Input: dimensioned drawing with shaded views. Units: mm. Origin: part minimum x, y, z. A direction names the side the tool comes from. Round coordinates to 2 decimals unless told otherwise and drop trailing zeros. Loops run counter-clockwise (first coordinate to the right, second up) from the corner with the lowest first, then second, coordinate; pieces in that order, holes last.
1) Draft query along Y for the marked faces 1, 2 and 3. Return one class per face: pulls with the +Y half, pulls with the -Y half, needs draft (parallel to the pull), parting line crosses it, or undercut.
2) Section D-D, the plane z = 13. Return loops of the section in (x, y).
3) Ray query, line 1 along Y through (x, z) = (25, 19); line 2 along Z through (x, y) = (17.5, 81); line 3 along Y through (x, z) = (26, 29.5). Return the intervals inside material, ascending.
4) First-contact query: pin 1 (8 mm diameter, centred on x = 24.5, y = 78, fed in from +Z); pin 2 (11 mm diameter, centred on x = 25, y = 35, fed in from +Z); pin 3 (8 mm diameter, centred on x = 21.5, y = 52.5, fed in from -Z); pin 4 (3.5 mm diameter, centred on x = 12.5, z = 3.5, fed in from +Y). Flat tips, straight axial feed; report the tip coordinate or a pass-through.
5) Section A-A, the plane x = 25. Return loops of the section in (y, z).
6) Section C-C, the plane x = 18.5. Return loops of the section in (y, z).
7) Section B-B, the plane y = 35. Return loops of the section in (x, z).
8) Access query for the marked faces 4, 5, 6 and 7. Directions: +Z, -Z, +X, -X, +Y, -Y. A direction counts if a zero-diameter tool reaches every point of the face in a straight line with its end or side. Return the directions, or none.
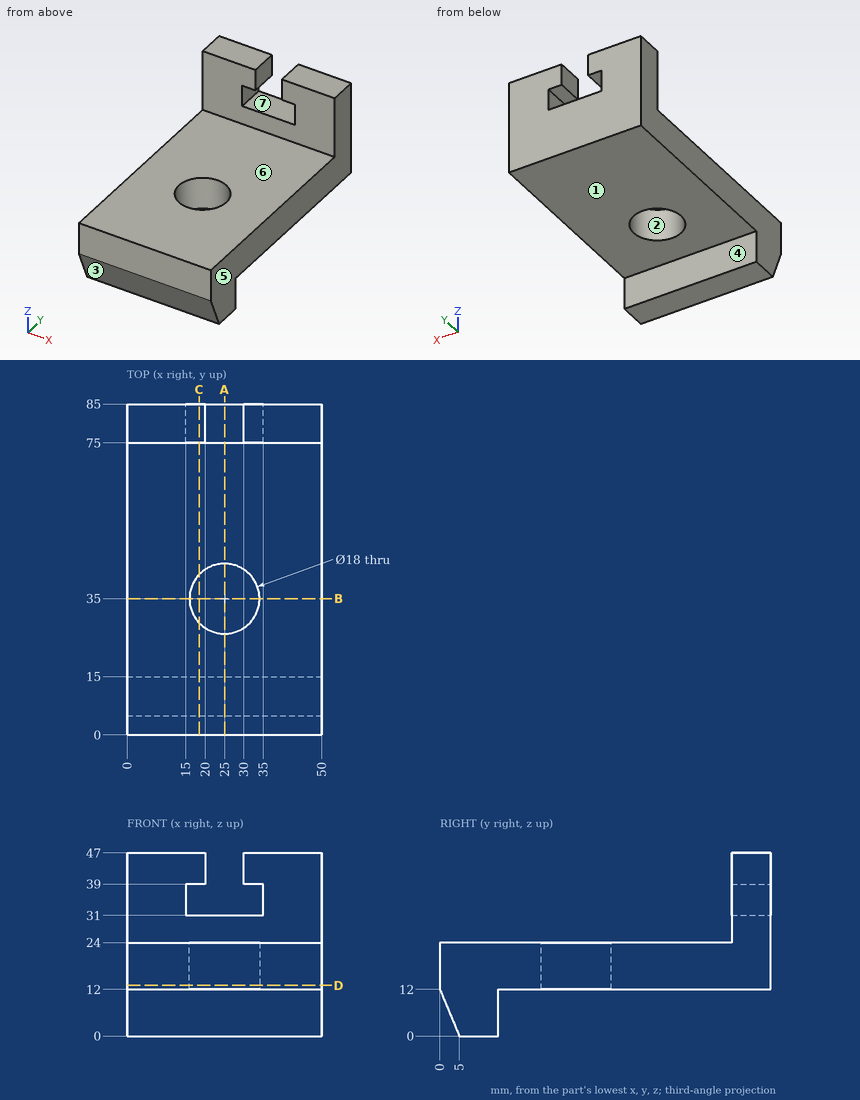
Final values:
1. face 1: needs draft
1. face 2: undercut
1. face 3: pulls with the -Y half
2. outline: (0, 0) - (50, 0) - (50, 85) - (0, 85) - close; hole circle Ø18 at (25, 35)
3. line 1: y = 0 to 26, 44 to 85
3. line 2: z = 12 to 31, 39 to 47
3. line 3: y = 75 to 85
4. pin 1: stops at z = 31
4. pin 2: passes through
4. pin 3: stops at z = 12
4. pin 4: stops at y = 15
5. outline: (0, 12) - (5, 0) - (15, 0) - (15, 12) - (26, 12) - (26, 24) - (0, 24) - close; (44, 12) - (85, 12) - (85, 31) - (75, 31) - (75, 24) - (44, 24) - close
6. outline: (0, 12) - (5, 0) - (15, 0) - (15, 12) - (28.78, 12) - (28.78, 24) - (0, 24) - close; (41.22, 12) - (85, 12) - (85, 31) - (75, 31) - (75, 24) - (41.22, 24) - close; (75, 39) - (85, 39) - (85, 47) - (75, 47) - close
7. outline: (0, 12) - (16, 12) - (16, 24) - (0, 24) - close; (34, 12) - (50, 12) - (50, 24) - (34, 24) - close
8. face 4: -Z, +X, -X, +Y
8. face 5: +Z, -Z, +X, +Y, -Y
8. face 6: +Z, +X, -X, -Y
8. face 7: +Y, -Y
